Verification items for the finished model (mm, model axes). Coordinates: 2 decimals unless noted, no trailing zeros. Write each loop counter-clockwise with the first axis right and the second up, starting at its lowest first coordinate (ties: lowest second). Pieces come first, ordered by that corner, then holes. Notation, with made-up numbers: (84, 71) - (116, 71) arc R23 cw to (116, 79) - close; hole circle Ø5 at (12, 77.25). An arc over 180 degrees is marked (long way). Use CSV: the item, a comma, the result in double quotes. Start each with the question number.
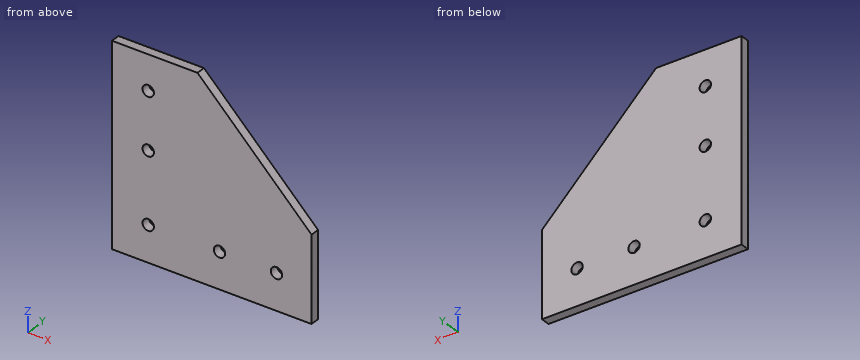
```python
from build123d import *

# Parameters (mm, degrees)
SKETCH2_W             = 70
SKETCH2_H             = 70
BOSS_EXTRUDE1_DEPTH   = 3.175
F_4_0MM_DOWEL_HOLE1_D = 4
CUT_EXTRUDE1_DEPTH    = 50.599199842


with BuildPart() as part:
    # Sketch2 → Boss-Extrude1 (new body)
    with BuildSketch(Plane(origin=(0, 0, 0), x_dir=(1, 0, 0), z_dir=(0, 1, 0))):
        Rectangle(SKETCH2_W, SKETCH2_H)
    extrude(amount=BOSS_EXTRUDE1_DEPTH)

    # Ø4.0mm Dowel Hole1 (through all)
    with Locations(Plane(origin=(0, 3.175, 0), x_dir=(1, 0, 0), z_dir=(0, 1, 0))):
        with Locations((-22.3, 22.3), (22.7, 22.3), (2.7, 22.3), (-22.3, -2.7), (-22.3, -22.7)):
            Hole(F_4_0MM_DOWEL_HOLE1_D / 2)

    # Sketch8 → Cut-Extrude1 (cut, through all)
    with BuildSketch(Plane(origin=(0, 3.175, 0), x_dir=(1, 0, 0), z_dir=(0, 1, 0))):
        Polygon((-5, -35), (35, 5), (35, -35), align=None)
    extrude(amount=-CUT_EXTRUDE1_DEPTH, mode=Mode.SUBTRACT)


solid = part.part
```
Q1. Cross-section at C-C (y = 2.2). Record the cut outline in (x, z).
Q2. Cross-section at A-A (z = 2.7). Record the cut outline in (x, y) (3 decimals).
Q3. Cross-section at B-B (x = 2.7). Record the cut outline in (y, z) (3 decimals), plus the area to 3 significant figures.
Q4. Gauge pin test, flat end, axial feed: pin 1 (1 mm diameter, centred on y = 0.5, z = 14.5, fed in from +X). Record the tip position at first contact, or that the pin passes through.
Q5. Cross-section at D-D (x = -22.3). Record the cut outline in (y, z) (3 decimals), plus the area to 3 significant figures.
Q6. Scan lines: line 1 along X through (y, z) = (1.5, -22.3); line 2 along X through (y, z) = (1, 22.7). Record each from-to range of solid material in increasing order. Write a range as from..to.
Reply:
1,outline,"(-35, -35) - (35, -35) - (35, -5) - (-5, 35) - (-35, 35) - close; hole circle Ø4 at (-22.3, -22.3); hole circle Ø4 at (-22.3, 2.7); hole circle Ø4 at (-22.3, 22.7); hole circle Ø4 at (2.7, -22.3); hole circle Ø4 at (22.7, -22.3)"
2,outline,"(-35, 0) - (-24.3, 0) - (-24.3, 3.175) - (-35, 3.175) - close; (-20.3, 0) - (27.3, 0) - (27.3, 3.175) - (-20.3, 3.175) - close"
3,outline,"(0, -35) - (3.175, -35) - (3.175, -24.3) - (0, -24.3) - close; (0, -20.3) - (3.175, -20.3) - (3.175, 27.3) - (0, 27.3) - close"
3,area,"185 mm^2"
4,pin 1,"x = 16"
5,outline,"(0, -35) - (3.175, -35) - (3.175, -24.3) - (0, -24.3) - close; (0, -20.3) - (3.175, -20.3) - (3.175, 0.7) - (0, 0.7) - close; (0, 4.7) - (3.175, 4.7) - (3.175, 20.7) - (0, 20.7) - close; (0, 24.7) - (3.175, 24.7) - (3.175, 35) - (0, 35) - close"
5,area,"184 mm^2"
6,line 1,"-35..-24.3, -20.3..0.7, 4.7..20.7, 24.7..35"
6,line 2,"-35..-24.3, -20.3..7.3"
